Work out the finished part from the listing and answer in its coordinate system (mm). A direction names the side the tool comes from. Give positions to 0.01 mm unless a question says otherwise; leave off trailing zeros. Order: outer loops, then holes, each group sorted by start corner. A loop starts at its lowest first (then second) coordinate and runs counter-clockwise, first axis right, second up. Notation, with made-up numbers: (51, 71) - (110, 71) arc R17 ccw to (110, 103) - close; hole circle Ø7 at (66.25, -33.5). An arc over 180 degrees is marked (long way). Put each result on its own line as item: value.
```python
from build123d import *

# Parameters (mm, degrees)
BOSS_EXTRUDE1_DEPTH             = 155
BOSS_EXTRUDE1_DEPTH_BACK        = 200
SKETCH1_R                       = 107.5
SKETCH1_R_2                     = 100
SKETCH1_3_R                     = 100
SKETCH1_3_R_2                   = 95
SKETCH1_3_R_3                   = 31
BOSS_EXTRUDE2_DEPTH             = 17
SKETCH1_5_R                     = 95
SKETCH1_5_R_2                   = 31
CUT_EXTRUDE1_DEPTH              = 4
F_4_0MM_DOWEL_HOLE1_D           = 4
F_4_0MM_DOWEL_HOLE1_CSINK_D     = 4.05
F_4_0MM_DOWEL_HOLE1_CSINK_ANGLE = 90
CUT_EXTRUDE2_DEPTH              = 5
SKETCH8_R                       = 200
SKETCH8_R_2                     = 100
BOSS_EXTRUDE3_DEPTH             = 5
F_4_0MM_DOWEL_HOLE2_D           = 4
F_4_0MM_DOWEL_HOLE2_CSINK_D     = 4.05
F_4_0MM_DOWEL_HOLE2_CSINK_ANGLE = 90
SKETCH12_R                      = 102.5
CUT_EXTRUDE3_DEPTH              = 2.5


with BuildPart() as part:
    # Sketch1 → Boss-Extrude1 (new, two sides: drawn at the far end of the back side and taken through both)
    with BuildSketch(Plane(origin=(0, 0, 0), x_dir=(1, 0, 0), z_dir=(0, 1, 0)).offset(-BOSS_EXTRUDE1_DEPTH_BACK)):
        with Locations(Location((0, 0, 0), (0, 0, 270))):
            Circle(SKETCH1_R)
        with Locations(Location((0, 0, 0), (0, 0, 270))):
            Circle(SKETCH1_R_2, mode=Mode.SUBTRACT)
    extrude(amount=BOSS_EXTRUDE1_DEPTH + BOSS_EXTRUDE1_DEPTH_BACK)

    # Sketch1<3> → Boss-Extrude2 (add)
    # profile 1 of 2: a face of its own
    with BuildSketch(Plane(origin=(0, 0, 0), x_dir=(1, 0, 0), z_dir=(0, 1, 0))):
        with Locations(Location((0, 0, 0), (0, 0, 270))):
            Circle(SKETCH1_3_R)
        Circle(SKETCH1_3_R_2, mode=Mode.SUBTRACT)
    # profile 2 of 2: a face of its own
    with BuildSketch(Plane(origin=(0, 0, 0), x_dir=(1, 0, 0), z_dir=(0, 1, 0))):
        Circle(SKETCH1_3_R_2)
        with Locations(Location((0, 0, 0), (0, 0, 270))):
            Circle(SKETCH1_3_R_3, mode=Mode.SUBTRACT)
    extrude(amount=-BOSS_EXTRUDE2_DEPTH)

    # Sketch1<5> → Cut-Extrude1 (cut)
    with BuildSketch(Plane(origin=(0, 0, 0), x_dir=(1, 0, 0), z_dir=(0, 1, 0))):
        with Locations(Location((0, 0, 0), (0, 0, 270))):
            Circle(SKETCH1_5_R)
        with Locations(Location((0, 0, 0), (0, 0, 270))):
            Circle(SKETCH1_5_R_2, mode=Mode.SUBTRACT)
    extrude(amount=-CUT_EXTRUDE1_DEPTH, mode=Mode.SUBTRACT)

    # Ø4.0mm Dowel Hole1 (through all)
    with Locations(Plane(origin=(0, -17, 0), x_dir=(-1, 0, 0), z_dir=(0, -1, 0))):
        with Locations((0, 70), (49.497474683, 49.497474683), (-49.497474683, 49.497474683), (-70, 0), (-49.497474683, -49.497474683), (0, -70), (49.497474683, -49.497474683), (70, 0)):
            CounterSinkHole(F_4_0MM_DOWEL_HOLE1_D / 2, F_4_0MM_DOWEL_HOLE1_CSINK_D / 2, counter_sink_angle=F_4_0MM_DOWEL_HOLE1_CSINK_ANGLE)

    # Sketch5 → Cut-Extrude2 (cut)
    with BuildSketch(Plane(origin=(0, -4, 0), x_dir=(1, 0, 0), z_dir=(0, 1, 0))):
        Polygon((46.231488359, 46.231488359), (50.692908646, 45.036054396), (53.95889497, 48.30204072), (52.763461007, 52.763461007), (48.30204072, 53.95889497), (45.036054396, 50.692908646), align=None)
        Polygon((0, 65.381197846), (4, 67.690598923), (4, 72.309401077), (0, 74.618802154), (-4, 72.309401077), (-4, 67.690598923), align=None)
        Polygon((65.381197846, 0), (67.690598923, -4), (72.309401077, -4), (74.618802154, 0), (72.309401077, 4), (67.690598923, 4), align=None)
        Polygon((46.231488359, -46.231488359), (45.036054396, -50.692908646), (48.30204072, -53.95889497), (52.763461007, -52.763461007), (53.95889497, -48.30204072), (50.692908646, -45.036054396), align=None)
        Polygon((0, -65.381197846), (-4, -67.690598923), (-4, -72.309401077), (0, -74.618802154), (4, -72.309401077), (4, -67.690598923), align=None)
        Polygon((-46.231488359, -46.231488359), (-50.692908646, -45.036054396), (-53.95889497, -48.30204072), (-52.763461007, -52.763461007), (-48.30204072, -53.95889497), (-45.036054396, -50.692908646), align=None)
        Polygon((-65.381197846, 0), (-67.690598923, 4), (-72.309401077, 4), (-74.618802154, 0), (-72.309401077, -4), (-67.690598923, -4), align=None)
        Polygon((-46.231488359, 46.231488359), (-45.036054396, 50.692908646), (-48.30204072, 53.95889497), (-52.763461007, 52.763461007), (-53.95889497, 48.30204072), (-50.692908646, 45.036054396), align=None)
    extrude(amount=-CUT_EXTRUDE2_DEPTH, mode=Mode.SUBTRACT)

    # Sketch8 → Boss-Extrude3 (add)
    with BuildSketch(Plane(origin=(0, -200, 0), x_dir=(-1, 0, 0), z_dir=(0, -1, 0))):
        with Locations(Location((0, 0, 0), (0, 0, 90))):
            Circle(SKETCH8_R)
        with Locations(Location((0, 0, 0), (0, 0, 270))):
            Circle(SKETCH8_R_2, mode=Mode.SUBTRACT)
    extrude(amount=-BOSS_EXTRUDE3_DEPTH)

    # Ø4.0mm Dowel Hole2 (through all)
    with Locations(Plane(origin=(0, -195, 0), x_dir=(1, 0, 0), z_dir=(0, 1, 0))):
        with Locations((160, 0), (113.13708499, 113.13708499), (0, 160), (-113.13708499, 113.13708499), (-160, 0), (-113.13708499, -113.13708499), (113.13708499, -113.13708499), (0, -160)):
            CounterSinkHole(F_4_0MM_DOWEL_HOLE2_D / 2, F_4_0MM_DOWEL_HOLE2_CSINK_D / 2, counter_sink_angle=F_4_0MM_DOWEL_HOLE2_CSINK_ANGLE)

    # Sketch12 → Cut-Extrude3 (cut)
    with BuildSketch(Plane(origin=(0, 150, 0), x_dir=(1, 0, 0), z_dir=(0, 1, 0))):
        with Locations(Location((0, 0, 0), (0, 0, 270))):
            Circle(SKETCH12_R)
    extrude(amount=CUT_EXTRUDE3_DEPTH, mode=Mode.SUBTRACT)


solid = part.part
```
(1) Section C-C, the plane z = -60 is taken. Write down the section's boundary in (x, y).
Geometry check:
outline: (-190.79, -200) - (-80, -200) - (-80, -17) - (80, -17) - (80, -200) - (190.79, -200) - (190.79, -195) - (89.2, -195) - (89.2, 155) - (80, 155) - (80, 152.5) - (83.1, 152.5) - (83.1, 150) - (80, 150) - (80, 0) - (73.65, 0) - (73.65, -4) - (-73.65, -4) - (-73.65, 0) - (-80, 0) - (-80, 150) - (-83.1, 150) - (-83.1, 152.5) - (-80, 152.5) - (-80, 155) - (-89.2, 155) - (-89.2, -195) - (-190.79, -195) - close
(2) Straight lines are drawn through the part: line 1 (X direction, y = -119, z = 2); line 2 (Y direction, x = -163, z = -60.5); line 3 (Y direction, x = 31, z = -22). For each, find the intervals that lie inside material, in ascending order.
Geometry check:
line 1: x = -107.48 to -99.98, 99.98 to 107.48
line 2: y = -200 to -195
line 3: y = -17 to -4
(3) Given pin 1 (3.5 mm diameter, centred on x = -160, z = 0, fed in from -Y); pin 2 (4 mm diameter, centred on x = -59, z = -28.5, fed in from +Y); pin 3 (2.5 mm diameter, centred on x = 70.5, y = -6, fed in from +Z); pin 4 (4 mm diameter, centred on y = 92, z = -70, fed in from +X), each flat-ended and moving along its own axis, determine where each tip first touches the part or whether it passes through.
Geometry check:
pin 1: passes through
pin 2: stops at y = -4
pin 3: stops at z = 82.22
pin 4: stops at x = 83.26
(4) Section B-B, the plane y = -97.5 is taken. Write down the section's boundary in (x, z).
Geometry check:
outline: circle Ø215 at (0, 0); hole circle Ø200 at (0, 0)
(5) A tool of negligible diameter and unlimited length cuts with its end or side. For faces 1 (the face through (60.075, -197.535, -190.764)), 2 (the face through (-92.74, -1.97, -20.59)), 3 (the face through (30.04, -109.78, 95.38)), 4 (the face through (-100.063, 151.232, -22.22)), from which of +Z, -Z, +X, -X, +Y, -Y can it reach the whole face along a straight path? Write none if from no direction.
Geometry check:
face 1: +Y, -Y
face 2: +Y
face 3: -Y
face 4: none
(6) Section A-A, the plane x = -89 is taken. Write down the section's boundary in (y, z), then the cut area to 3 significant figures.
Geometry check:
outline: (-200, -179.11) - (-195, -179.11) - (-195, -60.29) - (155, -60.29) - (155, -45.6) - (152.5, -45.6) - (152.5, -50.85) - (150, -50.85) - (150, -45.6) - (0, -45.6) - (0, -33.23) - (-4, -33.23) - (-4, 33.23) - (0, 33.23) - (0, 45.6) - (150, 45.6) - (150, 50.85) - (152.5, 50.85) - (152.5, 45.6) - (155, 45.6) - (155, 60.29) - (-195, 60.29) - (-195, 179.11) - (-200, 179.11) - (-200, 45.6) - (-17, 45.6) - (-17, -45.6) - (-200, -45.6) - close
area: 12,900 mm²
(7) Section D-D, the plane z = -137.5 is taken. Write down the section's boundary in (x, y).
Geometry check:
outline: (-145.24, -200) - (145.24, -200) - (145.24, -195) - (-145.24, -195) - close
(8) Determine the mould class of faces 5 (the face through (-86, -195, -86)), 6 (the face through (92, -200, -42)), 7 (the face through (-22, 152.5, 98)) for opening direction Y: pulls with the +Y half, pulls with the -Y half, needs draft (parallel to the pull), parting line crosses it, or undercut.
Geometry check:
face 5: pulls with the +Y half
face 6: pulls with the -Y half
face 7: undercut
